```python
from build123d import *

# Parameters (mm, degrees)
SKETCH1_R                                       = 6
BOSS_EXTRUDE1_DEPTH                             = 4
CSK_FOR_M2_FLAT_HEAD_MACHINE_SCREW1_D           = 2.6
CSK_FOR_M2_FLAT_HEAD_MACHINE_SCREW1_CSINK_D     = 4.4
CSK_FOR_M2_FLAT_HEAD_MACHINE_SCREW1_CSINK_ANGLE = 90


with BuildPart() as part:
    # Sketch1 → Boss-Extrude1 (new body)
    with BuildSketch(Plane(origin=(0, 0, 0), x_dir=(1, 0, 0), z_dir=(0, 1, 0))):
        with BuildLine():
            Line((-2.5, -12.951833847), (-2.5, -38.5))
            Line((-2.5, -38.5), (2.5, -38.5))
            Line((2.5, -38.5), (2.5, -12.951833847))
            ThreePointArc((2.5, -12.951833847), (3.295532486, -9.043154047), (5.555555556, -5.756370599))
            ThreePointArc((5.555555556, -5.756370599), (0, 8), (-5.555555556, -5.756370599))
            ThreePointArc((-5.555555556, -5.756370599), (-3.295532486, -9.043154047), (-2.5, -12.951833847))
        make_face()
        Circle(SKETCH1_R, mode=Mode.SUBTRACT)
    extrude(amount=BOSS_EXTRUDE1_DEPTH)

    # CSK for M2 Flat Head Machine Screw1 (through all)
    with Locations(Plane(origin=(0, 0, 0), x_dir=(-1, 0, 0), z_dir=(0, -1, 0))):
        with Locations((0, -23.5), (0, -33.5)):
            CounterSinkHole(CSK_FOR_M2_FLAT_HEAD_MACHINE_SCREW1_D / 2, CSK_FOR_M2_FLAT_HEAD_MACHINE_SCREW1_CSINK_D / 2, counter_sink_angle=CSK_FOR_M2_FLAT_HEAD_MACHINE_SCREW1_CSINK_ANGLE)


solid = part.part
```
Could you check a few things on this model? Use its own coordinates, in mm. A direction names the side the tool comes from. Give positions to 0.01 mm unless a question says otherwise; leave off trailing zeros. Loops run counter-clockwise (first coordinate to the right, second up) from the corner with the lowest first, then second, coordinate; pieces in that order, holes last. Notation, with made-up numbers: (67.5, 38) - (114.5, 38) arc R30 cw to (114.5, 62) - close; hole circle Ø8 at (38, 33.25). An arc over 180 degrees is marked (long way). Use one line per item in the form item = value.
1. I want a section at B-B (y = 3.3). Please give me the cut outline in (x, z).
Response values:
outline = (-5.56, 5.76) arc R8 ccw (long way) to (5.56, 5.76) arc R10 cw to (2.5, 12.95) - (2.5, 38.5) - (-2.5, 38.5) - (-2.5, 12.95) arc R10 cw to start; hole circle Ø12 at (0, 0); hole circle Ø2.6 at (0, 23.5); hole circle Ø2.6 at (0, 33.5)
2. I want a section at D-D (x = 4.5). Please give me the cut outline in (y, z).
Response values:
outline = (0, -6.61) - (4, -6.61) - (4, -3.97) - (0, -3.97) - close; (0, 3.97) - (4, 3.97) - (4, 6.95) - (0, 6.95) - close
3. Thinking about a two-plate mould opening in Z: for faces 3 (the face through (-2.5, 2, 26)), 4 (the face through (-0.17, 2.47, 32.21)), 5 (the face through (0, 2, -8)), which applies, released by +Z, released by -Z, zero draft, split by the parting line, or undercut?
Response values:
face_3 = zero draft
face_4 = undercut
face_5 = split by the parting line
4. I want a section at C-C (x = 0). Please give me the cut outline in (y, z).
Response values:
outline = (0, -8) - (4, -8) - (4, -6) - (0, -6) - close; (0, 6) - (4, 6) - (4, 22.2) - (0.9, 22.2) - (0, 21.3) - close; (0, 25.7) - (0.9, 24.8) - (4, 24.8) - (4, 32.2) - (0.9, 32.2) - (0, 31.3) - close; (0, 35.7) - (0.9, 34.8) - (4, 34.8) - (4, 38.5) - (0, 38.5) - close
5. I need wall thicknesses on probe 1 along Z at (x, y) = (0, 1.6); probe 2 along X at (y, z) = (2.8, 23.5); probe 3 along X at (y, z) = (2.45, 0). Which ranges of each line are inside material? Lowest first, please.
Response values:
probe_1 = -8 to -6, 6 to 22.2, 24.8 to 32.2, 34.8 to 38.5
probe_2 = -2.5 to -1.3, 1.3 to 2.5
probe_3 = -8 to -6, 6 to 8
6. I'm going to push flat-ended pins straight in: pin 1 Ø1.5 at (y, z) = (2, 31.5) entering from +X; pin 2 Ø1 at (x, y) = (5.5, 2.5) entering from -Z (3 decimals); pin 3 Ø2.5 at (x, z) = (0, 33.5) entering from -Y. Where does each tip first touch, or does it pass through?
Response values:
pin_1 = 2.5
pin_2 = -6.245
pin_3 = through
7. I want a section at A-A (z = 33.5). Please give me the cut outline in (x, y), and give its area (3 significant figures).
Response values:
outline = (-2.5, 0) - (-2.2, 0) - (-1.3, 0.9) - (-1.3, 4) - (-2.5, 4) - close; (1.3, 0.9) - (2.2, 0) - (2.5, 0) - (2.5, 4) - (1.3, 4) - close
area = 8.79 mm²
8. On a 3-axis mill with a long thin cutter (end or side, diameter ignored), from which of +Z, -Z, +X, -X, +Y, -Y can I reach the whole of each face in a straight line? I mean faces 1 (the face through (1, 0, 13)), 2 (the face through (2.5, 2, 26)). Say none if no direction works.
Response values:
face_1 = +Z, -Z, +X, -X, -Y
face_2 = +Z, +X, +Y, -Y
